```python
from build123d import *

# Parameters (mm, degrees)
SKETCH1_R           = 10
BOSS_EXTRUDE1_DEPTH = 6
BOSS_EXTRUDE2_START = -18
SKETCH1_2_R         = 10
BOSS_EXTRUDE2_DEPTH = 6
SKETCH4_W           = 20
SKETCH4_H           = 24
BOSS_EXTRUDE3_DEPTH = 29


with BuildPart() as part:
    # Sketch1 → Boss-Extrude1 (new body)
    with BuildSketch(Plane.XY):
        with BuildLine():
            Line((40, -14.5), (-40, -14.5))
            ThreePointArc((-40, -14.5), (-54.5, 0), (-40, 14.5))
            Line((-40, 14.5), (40, 14.5))
            ThreePointArc((40, 14.5), (54.5, 0), (40, -14.5))
        make_face()
        with Locations((-40, 0)):
            Circle(SKETCH1_R, mode=Mode.SUBTRACT)
        with Locations((40, 0)):
            Circle(SKETCH1_R, mode=Mode.SUBTRACT)
    extrude(amount=BOSS_EXTRUDE1_DEPTH)



with BuildPart() as body_2:
    # Sketch1_2 → Boss-Extrude2 (new body)
    with BuildSketch(Plane.XY.offset(BOSS_EXTRUDE2_START)):
        with BuildLine():
            Line((40, -14.5), (-40, -14.5))
            ThreePointArc((-40, -14.5), (-54.5, 0), (-40, 14.5))
            Line((-40, 14.5), (40, 14.5))
            ThreePointArc((40, 14.5), (54.5, 0), (40, -14.5))
        make_face()
        with Locations((-40, 0)):
            Circle(SKETCH1_2_R, mode=Mode.SUBTRACT)
        with Locations((40, 0)):
            Circle(SKETCH1_2_R, mode=Mode.SUBTRACT)
    extrude(amount=BOSS_EXTRUDE2_DEPTH)


with BuildPart() as part_1:
    add(part.part)

    add(body_2.part)  # Boss-Extrude3 merges body 2
    # Sketch4 → Boss-Extrude3 (add)
    with BuildSketch(Plane(origin=(0, 14.5, 0), x_dir=(1, 0, 0), z_dir=(0, 1, 0))):
        with Locations((0, 6)):
            Rectangle(SKETCH4_W, SKETCH4_H)
    extrude(amount=-BOSS_EXTRUDE3_DEPTH)


solid = part_1.part
```
Verification items for the finished model (mm, model axes). A direction names the side the tool comes from. Coordinates: 2 decimals unless noted, no trailing zeros. Order: outer loops, then holes, each group sorted by start corner. A loop starts at its lowest first (then second) coordinate and runs counter-clockwise, first axis right, second up. Notation, with made-up numbers: (83, -6) -> (89, -6) arc R6 ccw to (89, -2) -> close; hole circle Ø6 at (-36, 56.25). An arc over 180 degrees is marked (long way). Answer as CSV lines item,"result". Start each with the question number.
1) Set-up check for faces 5 (the face through (-10, 0, -6)), 6 (the face through (10, 0, -6)), 7 (the face through (-54.496, -0.319, 2.958)): record each of +Z, -Z, +X, -X, +Y, -Y from which the full face is reachable in a straight line by a thin tool's end or side.
2) Cross-section at B-B, the plane x = -17.5. Record the boundary of the cut face in (y, z), then the cut area to 3 significant figures.
3) Cross-section at A-A, the plane y = 0. Record the boundary of the cut face in (x, z).
4) Cross-section at C-C, the plane z = -16.5. Record the boundary of the cut face in (x, y), then the cut area to 3 significant figures.
5) Cross-section at D-D, the plane x = 41. Record the boundary of the cut face in (y, z), then the cut area to 3 significant figures.
6) Gauge pin test, flat ends, axial feed: pin 1 Ø1.5 at (y, z) = (-11, 1) entering from +X; pin 2 Ø2 at (y, z) = (-10, 3) entering from -X; pin 3 Ø10 at (y, z) = (-6, 2.5) entering from +X; pin 4 Ø5 at (x, z) = (-20, -4.5) entering from -Y. Record the tip position at first contact, or that the pin passes through.
7) Release check for a two-part mould opening along Y. For faces 1 (the face through (1, -14.5, -6)), 2 (the face through (28, 0, 0)), 3 (the face through (54.496, 0.319, 2.958)), 4 (the face through (-50, 0, -15)) record: released by +Y, released by -Y, zero draft, split by the parting line, or undercut.
8) Material ranges on L1, parallel to Z at x = -18.5, y = -6.25; L2, parallel to X at y = -7, z = -12.25; L3, parallel to Y at x = 40, z = -13.65, recorded low to high. Write a range as [from, to].
Conclusion:
1,face 5,"-X, +Y, -Y"
1,face 6,"+X, +Y, -Y"
1,face 7,"+Z, -Z, -X"
2,outline,"(-14.5, -18) -> (14.5, -18) -> (14.5, -12) -> (-14.5, -12) -> close; (-14.5, 0) -> (14.5, 0) -> (14.5, 6) -> (-14.5, 6) -> close"
2,area,"348 mm²"
3,outline,"(-54.5, -18) -> (-50, -18) -> (-50, -12) -> (-54.5, -12) -> close; (-54.5, 0) -> (-50, 0) -> (-50, 6) -> (-54.5, 6) -> close; (-30, -18) -> (30, -18) -> (30, -12) -> (10, -12) -> (10, 0) -> (30, 0) -> (30, 6) -> (-30, 6) -> (-30, 0) -> (-10, 0) -> (-10, -12) -> (-30, -12) -> close; (50, -18) -> (54.5, -18) -> (54.5, -12) -> (50, -12) -> close; (50, 0) -> (54.5, 0) -> (54.5, 6) -> (50, 6) -> close"
4,outline,"(-40, -14.5) -> (40, -14.5) arc R14.5 ccw to (40, 14.5) -> (-40, 14.5) arc R14.5 ccw to start; hole circle Ø20 at (-40, 0); hole circle Ø20 at (40, 0)"
4,area,"2,350 mm²"
5,outline,"(-14.47, -18) -> (-9.95, -18) -> (-9.95, -12) -> (-14.47, -12) -> close; (-14.47, 0) -> (-9.95, 0) -> (-9.95, 6) -> (-14.47, 6) -> close; (9.95, -18) -> (14.47, -18) -> (14.47, -12) -> (9.95, -12) -> close; (9.95, 0) -> (14.47, 0) -> (14.47, 6) -> (9.95, 6) -> close"
5,area,"108 mm²"
6,pin 1,"stops at x = 50.26"
6,pin 2,"stops at x = -51.37"
6,pin 3,"stops at x = 54.47"
6,pin 4,"passes through"
7,face 1,"released by -Y"
7,face 2,"zero draft"
7,face 3,"split by the parting line"
7,face 4,"undercut"
8,L1,"z = [-18, -12], [0, 6]"
8,L2,"x = [-52.7, -47.14], [-32.86, 32.86], [47.14, 52.7]"
8,L3,"y = [-14.5, -10], [10, 14.5]"
